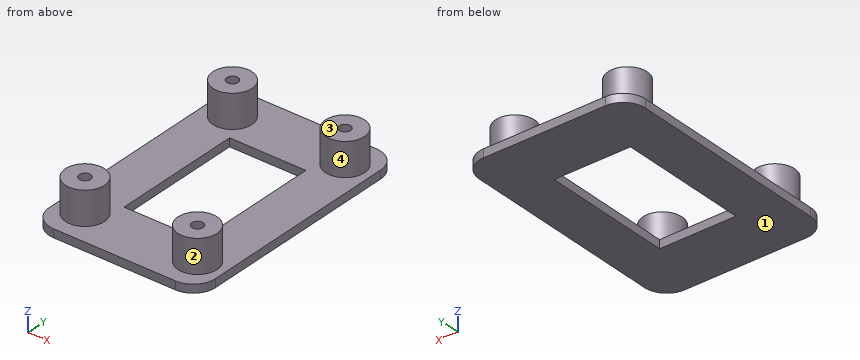
```python
from build123d import *

# Parameters (mm, degrees)
F1_DEPTH = 1.5
F2_R     = 3.525
F2_R_2   = 1.025
F3_DEPTH = 6
F4_W     = 13.78999
F4_H     = 23.601498
F5_DEPTH = 2


with BuildPart() as f1:
    # F0 (on Top) → F1 (new body)
    with BuildSketch(Plane.XY):
        with BuildLine():
            Line((11, 22.5), (-11, 22.5))
            ThreePointArc((-11, 22.5), (-13.828427, 21.328427), (-15, 18.5))
            Line((-15, 18.5), (-15, -18.5))
            ThreePointArc((-15, -18.5), (-13.828427, -21.328427), (-11, -22.5))
            Line((-11, -22.5), (11, -22.5))
            ThreePointArc((11, -22.5), (13.828427, -21.328427), (15, -18.5))
            Line((15, -18.5), (15, 18.5))
            ThreePointArc((15, 18.5), (13.828427, 21.328427), (11, 22.5))
        make_face()
    extrude(amount=F1_DEPTH)

    # F2 (on face) → F3 (join)
    with BuildSketch(Plane.XY.offset(1.5)):
        with Locations((-10.16, 16.51)):
            Circle(F2_R)
        with Locations((-10.16, 16.51)):
            Circle(F2_R_2, mode=Mode.SUBTRACT)
        with Locations((10.16, 16.51)):
            Circle(F2_R)
        with Locations((10.16, 16.51)):
            Circle(F2_R_2, mode=Mode.SUBTRACT)
        with Locations((-10.16, -16.51)):
            Circle(F2_R)
        with Locations((-10.16, -16.51)):
            Circle(F2_R_2, mode=Mode.SUBTRACT)
        with Locations((10.16, -16.51)):
            Circle(F2_R)
        with Locations((10.16, -16.51)):
            Circle(F2_R_2, mode=Mode.SUBTRACT)
    extrude(amount=F3_DEPTH)

    # F4 (on face) → F5 (cut)
    with BuildSketch(Plane.XY.offset(1.5)):
        Rectangle(F4_W, F4_H)
    extrude(amount=-F5_DEPTH, mode=Mode.SUBTRACT)


solid = f1.part
```
The listing builds one solid part. Answer for the finished solid, in the listing's coordinates (mm). Face numbers are marked on the shaded views. A direction names the side the tool comes from. Coordinates: 2 decimals unless noted, no trailing zeros. Loops run counter-clockwise (first coordinate to the right, second up) from the corner with the lowest first, then second, coordinate; pieces in that order, holes last. Notation, with made-up numbers: (70.5, 11.5) -> (113.5, 11.5) arc R19 cw to (113.5, 29.5) -> close; hole circle Ø7 at (78.5, 67.5). An arc over 180 degrees is marked (long way). Return JSON: item names as keys, results as strings. Group by question number.
(1) Which of the six approach directions +Z, -Z, +X, -X, +Y, -Y give full straight-line access (tool end or side, diameter ignored) to the marked faces 3 and 4?
(2) Determine the mould class of the marked faces 1 and 2 for opening direction X: released by +X, released by -X, zero draft, split by the parting line, or undercut.
(3) Find the intervals of material crossed by probe 1 along Y at (x, z) = (10.16, 3.1) (3 decimals); probe 2 along Y at (x, z) = (9.25, 5.25); probe 3 along Z at (x, y) = (-3, 20.5), in increasing order. Write a range as from..to.
(4) A cutting plane is placed at C-C on z = 3.5. Write down the section's boundary in (x, y) (3 decimals), and give its area (3 significant figures).
(5) A cutting plane is placed at B-B on y = 9. Write down the section's boundary in (x, z) (3 decimals).
(6) Given pin 1 Ø1.6 at (x, y) = (10.16, -16.51) entering from +Z, flat-ended and moving along its own axis, determine where the tip first touches the part or whether it passes through.
(7) A cutting plane is placed at A-A on x = -2.75. Write down the section's boundary in (y, z).
(8) A cutting plane is placed at D-D on y = 16.51. Write down the section's boundary in (x, z) (3 decimals).
The answers:
{
 "1": {"face 3": "+Z, +X, -X, +Y, -Y", "face 4": "+Z"},
 "2": {"face 1": "zero draft", "face 2": "undercut"},
 "3": {"probe 1": "y = -20.035..-17.535, -15.485..-12.985, 12.985..15.485, 17.535..20.035", "probe 2": "y = -19.92..-16.98, -16.04..-13.1, 13.1..16.04, 16.98..19.92", "probe 3": "z = 0..1.5"},
 "4": {"outline": "circle Ø7.05 at (-10.16, -16.51); circle Ø7.05 at (-10.16, 16.51); circle Ø7.05 at (10.16, -16.51); circle Ø7.05 at (10.16, 16.51); hole circle Ø2.05 at (-10.16, -16.51); hole circle Ø2.05 at (-10.16, 16.51); hole circle Ø2.05 at (10.16, -16.51); hole circle Ø2.05 at (10.16, 16.51)", "area": "143 mm^2"},
 "5": {"outline": "(-15, 0) -> (-6.895, 0) -> (-6.895, 1.5) -> (-15, 1.5) -> close; (6.895, 0) -> (15, 0) -> (15, 1.5) -> (6.895, 1.5) -> close"},
 "6": {"pin 1": "stops at z = 1.5"},
 "7": {"outline": "(-22.5, 0) -> (-11.8, 0) -> (-11.8, 1.5) -> (-22.5, 1.5) -> close; (11.8, 0) -> (22.5, 0) -> (22.5, 1.5) -> (11.8, 1.5) -> close"},
 "8": {"outline": "(-15, 0) -> (15, 0) -> (15, 1.5) -> (13.685, 1.5) -> (13.685, 7.5) -> (11.185, 7.5) -> (11.185, 1.5) -> (9.135, 1.5) -> (9.135, 7.5) -> (6.635, 7.5) -> (6.635, 1.5) -> (-6.635, 1.5) -> (-6.635, 7.5) -> (-9.135, 7.5) -> (-9.135, 1.5) -> (-11.185, 1.5) -> (-11.185, 7.5) -> (-13.685, 7.5) -> (-13.685, 1.5) -> (-15, 1.5) -> close"}
}
